Part model, mm, in its own coordinate system. A direction names the side the tool comes from. Coordinates: 2 decimals unless noted, no trailing zeros. Order: outer loops, then holes, each group sorted by start corner. A loop starts at its lowest first (then second) coordinate and runs counter-clockwise, first axis right, second up. Notation, with made-up numbers: (42, 16) - (74, 16) arc R24 ccw to (74, 28) - close; hole circle Ø5 at (-4, 12). An arc over 180 degrees is marked (long way). Use a Markdown table: item, result. Add a question column.
1) Tool access for faces 4 (the face through (0, -2.35, 2)), 5 (the face through (-14.1, 0, 2)): list every direction of +Z, -Z, +X, -X, +Y, -Y with a clear straight run to the whole face (end or side of a thin tool).
2) Saw through at A-A on y = -0.25. List the corners of the cut face in (x, z), then the cut area to 3 significant figures.
3) Wall check: L1, parallel to Y at x = -12, z = 3.05; L2, parallel to X at y = 0.5, z = 1.95; L3, parallel to X at y = -1.5, z = 0.5. Give the ranges that are in metal, low to high. Write a range as [from, to].
4) Saw through at B-B on x = 12. List the corners of the cut face in (y, z), then the cut area to 3 significant figures.
5) Saw through at D-D on x = -8.5. List the corners of the cut face in (y, z), then the cut area to 3 significant figures.
6) Drop flat-ended pins along their axis: P1, Ø2.5, axis at x = -12, y = -0.25, coming from the -Z side; P2, Ø2.5, axis at x = 1, z = 1.5, coming from the -Y side. Give the stop position or say it passes through.
7) Saw through at C-C on z = 3.6. List the corners of the cut face in (x, y).
8) Two-plate mould, pull along Y, no slides. Class faces 1 (the face through (11.98, -2.85, 2.33)), 2 (the face through (-13.5, -0.2, 2.3)), 3 (the face through (14.1, 0, 2)): +Y half, -Y half, draft (parallel to the pull), parting line (faces both ways), or undercut.
```python
from build123d import *

# Parameters (mm, degrees)
SKETCH_W       = 28.2
SKETCH_H       = 4.7
SKETCH_R       = 1.5
PAD_DEPTH      = 4.6
PAD001_DEPTH   = 4.6
PAD001_FACE2_W = 28.2
PAD001_FACE2_H = 4.6
PAD002_DEPTH   = 1


with BuildPart() as part:
    # Sketch → Pad (new body)
    with BuildSketch(Plane.XY):
        Rectangle(SKETCH_W, SKETCH_H)
        with Locations((-12, -0.25)):
            Circle(SKETCH_R, mode=Mode.SUBTRACT)
        with Locations((12, -0.25)):
            Circle(SKETCH_R, mode=Mode.SUBTRACT)
    extrude(amount=PAD_DEPTH)

    # Sketch001 (on Face8 of Pad) → Pad001 (join)
    with BuildSketch(Plane.XY.offset(4.6)):
        with BuildLine():
            ThreePointArc((10.467029, -2.35), (12, -2.85), (13.532971, -2.35))
            Line((10.467029, -2.35), (13.532971, -2.35))
        make_face()
        with BuildLine():
            ThreePointArc((-13.532971, -2.35), (-12, -2.85), (-10.467029, -2.35))
            Line((-13.532971, -2.35), (-10.467029, -2.35))
        make_face()
    extrude(amount=-PAD001_DEPTH)

    # Pad001 Face2 → Pad002 (add)
    with BuildSketch(Plane(origin=(0, 2.35, 2.3), x_dir=(1, 0, 0), z_dir=(0, 1, 0))):
        Rectangle(PAD001_FACE2_W, PAD001_FACE2_H)
    extrude(amount=PAD002_DEPTH)


solid = part.part
```
Results are:
| question | item | result |
|---|---|---|
| 1 | face 4 | +Z, -Z, -Y |
| 1 | face 5 | +Z, -Z, -X, +Y, -Y |
| 2 | outline | (-14.1, 0) - (-13.5, 0) - (-13.5, 4.6) - (-14.1, 4.6) - close; (-10.5, 0) - (10.5, 0) - (10.5, 4.6) - (-10.5, 4.6) - close; (13.5, 0) - (14.1, 0) - (14.1, 4.6) - (13.5, 4.6) - close |
| 2 | area | 102 mm2 |
| 3 | L1 | [-2.85, -1.75], [1.25, 3.35] |
| 3 | L2 | [-14.1, -13.3], [-10.7, 10.7], [13.3, 14.1] |
| 3 | L3 | [-14.1, -12.83], [-11.17, 11.17], [12.83, 14.1] |
| 4 | outline | (-2.85, 0) - (-1.75, 0) - (-1.75, 4.6) - (-2.85, 4.6) - close; (1.25, 0) - (3.35, 0) - (3.35, 4.6) - (1.25, 4.6) - close |
| 4 | area | 14.7 mm2 |
| 5 | outline | (-2.35, 0) - (3.35, 0) - (3.35, 4.6) - (-2.35, 4.6) - close |
| 5 | area | 26.2 mm2 |
| 6 | P1 | through |
| 6 | P2 | y = -2.35 |
| 7 | outline | (-14.1, -2.35) - (-13.53, -2.35) arc R2.6 ccw to (-10.47, -2.35) - (10.47, -2.35) arc R2.6 ccw to (13.53, -2.35) - (14.1, -2.35) - (14.1, 3.35) - (-14.1, 3.35) - close; hole circle Ø3 at (-12, -0.25); hole circle Ø3 at (12, -0.25) |
| 8 | face 1 | -Y half |
| 8 | face 2 | undercut |
| 8 | face 3 | draft |
